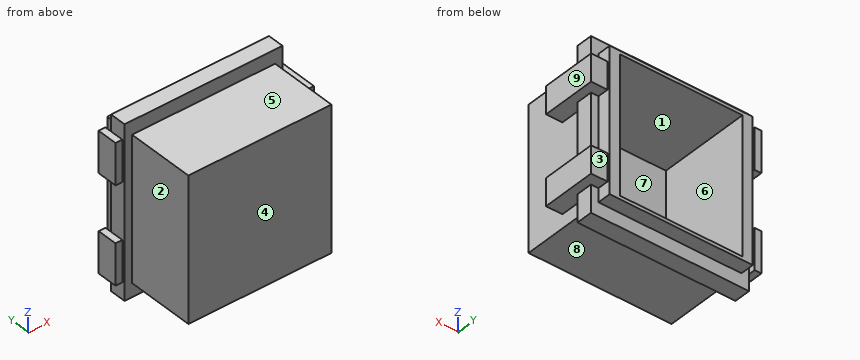
from build123d import *

# Parameters (mm, degrees)
SKETCH1_W           = 133.35
SKETCH1_H           = 133.35
BOSS_EXTRUDE1_DEPTH = 63.5
SKETCH2_W           = 147.32
SKETCH2_H           = 158.75
BOSS_EXTRUDE2_DEPTH = 15.24
SKETCH3_W           = 133.35
SKETCH3_H           = 133.35
BOSS_EXTRUDE3_DEPTH = 12.7
SKETCH4_W           = 38.1
SKETCH4_H           = 19.05
BOSS_EXTRUDE4_DEPTH = 6.35
SKETCH5_W           = 25.4
SKETCH5_H           = 50.8
BOSS_EXTRUDE5_DEPTH = 15.24
SKETCH7_W           = 114.3
SKETCH7_H           = 127
CUT_EXTRUDE1_DEPTH  = 86.36


with BuildPart() as part:
    # Sketch1 → Boss-Extrude1 (new body)
    with BuildSketch(Plane(origin=(0, 0, 0), x_dir=(1, 0, 0), z_dir=(0, 1, 0))):
        Rectangle(SKETCH1_W, SKETCH1_H)
    extrude(amount=BOSS_EXTRUDE1_DEPTH)

    # Sketch2 → Boss-Extrude2 (add)
    with BuildSketch(Plane(origin=(0, 63.5, 0), x_dir=(1, 0, 0), z_dir=(0, 1, 0))):
        Rectangle(SKETCH2_W, SKETCH2_H)
    extrude(amount=BOSS_EXTRUDE2_DEPTH)

    # Sketch3 → Boss-Extrude3 (add)
    with BuildSketch(Plane(origin=(0, 78.74, 0), x_dir=(1, 0, 0), z_dir=(0, 1, 0))):
        Rectangle(SKETCH3_W, SKETCH3_H)
    extrude(amount=BOSS_EXTRUDE3_DEPTH)

    # Sketch4 → Boss-Extrude4 (add)
    with BuildSketch(Plane.ZY.offset(73.66)):
        with Locations((45.085, 75.565)):
            Rectangle(SKETCH4_W, SKETCH4_H)
    boss_extrude4 = extrude(amount=BOSS_EXTRUDE4_DEPTH)

    # Mirror1: Boss-Extrude4 across plane
    add(boss_extrude4.mirror(Plane.XY))

    # Sketch5 → Boss-Extrude5 (add)
    with BuildSketch(Plane(origin=(66.675, 0, 0), x_dir=(0, 0, -1), z_dir=(1, 0, 0))):
        with Locations((-41.275, 63.5)):
            Rectangle(SKETCH5_W, SKETCH5_H)
    boss_extrude5 = extrude(amount=BOSS_EXTRUDE5_DEPTH)

    # Mirror2: Boss-Extrude5 across plane
    add(boss_extrude5.mirror(Plane.XY))

    # Sketch7 → Cut-Extrude1 (cut)
    with BuildSketch(Plane(origin=(0, 91.44, 0), x_dir=(1, 0, 0), z_dir=(0, 1, 0))):
        Rectangle(SKETCH7_W, SKETCH7_H)
    extrude(amount=-CUT_EXTRUDE1_DEPTH, mode=Mode.SUBTRACT)


solid = part.part
CAD build for the part. Positions are in the model's coordinates, mm. Face numbers are marked on the shaded views. A direction names the side the tool comes from. Coordinates: 2 decimals unless noted, no trailing zeros. Order: outer loops, then holes, each group sorted by start corner. A loop starts at its lowest first (then second) coordinate and runs counter-clockwise, first axis right, second up.
Item 1: Two-plate mould, pull along Z, no slides. Class the marked faces 6, 7, 8 and 9: +Z half, -Z half, draft (parallel to the pull), parting line (faces both ways), or undercut.
Check sheet entries:
face 6: undercut
face 7: undercut
face 8: -Z half
face 9: draft
Item 2: 3-axis set-ups, long thin cutter, end or side, ignore diameter. For the marked faces 1, 2, 3, 4 and 5: which of +Z, -Z, +X, -X, +Y, -Y reach the whole face in a straight line?
Check sheet entries:
face 1: +Y
face 2: +Z, -Z, -X, -Y
face 3: +Z, -Z, +X, +Y
face 4: +Z, -Z, +X, -X, -Y
face 5: +Z, +X, -X, -Y
Item 3: Drill centre lines: L1, parallel to X at y = 18.5, z = -17 (3 decimals); L2, parallel to X at y = 44.5, z = 40 (3 decimals); L3, parallel to Z at x = 53.5, y = 63 (3 decimals). Where is each one in solid material? Low to high.
Check sheet entries:
L1: x = -66.675 to -57.15, 57.15 to 66.675
L2: x = -66.675 to -57.15, 57.15 to 81.915
L3: z = -66.675 to -63.5, 63.5 to 66.675
Item 4: Pin check, flat tips, straight feed: pin 1 Ø2 at (x, z) = (69, -2) entering from -Y; pin 2 Ø5 at (x, y) = (-22, 18.5) entering from +Z (3 decimals); pin 3 Ø3 at (x, y) = (-18.5, 53.5) entering from -Z (3 decimals). Stop position of each tip, or through.
Check sheet entries:
pin 1: stops at y = 63.5
pin 2: stops at z = 66.675
pin 3: stops at z = -66.675
Item 5: Band-saw the part on D-D on z = -3. List the corners of the cut face in (x, y) (3 decimals), plus the area to 3 significant figures.
Check sheet entries:
outline: (-73.66, 63.5) - (-66.675, 63.5) - (-66.675, 0) - (66.675, 0) - (66.675, 63.5) - (73.66, 63.5) - (73.66, 78.74) - (66.675, 78.74) - (66.675, 91.44) - (57.15, 91.44) - (57.15, 5.08) - (-57.15, 5.08) - (-57.15, 91.44) - (-66.675, 91.44) - (-66.675, 78.74) - (-73.66, 78.74) - close
area: 2,540 mm2
Item 6: Band-saw the part on A-A on y = 13.5. List the corners of the cut face in (x, z) (3 decimals), plus the area to 3 significant figures.
Check sheet entries:
outline: (-66.675, -66.675) - (66.675, -66.675) - (66.675, 66.675) - (-66.675, 66.675) - close; hole (-57.15, -63.5) - (57.15, -63.5) - (57.15, 63.5) - (-57.15, 63.5) - close
area: 3,270 mm2
Item 7: Band-saw the part on B-B on z = 39. List the corners of the cut face in (x, y) (3 decimals).
Check sheet entries:
outline: (-80.01, 66.04) - (-73.66, 66.04) - (-73.66, 63.5) - (-66.675, 63.5) - (-66.675, 0) - (66.675, 0) - (66.675, 38.1) - (81.915, 38.1) - (81.915, 88.9) - (66.675, 88.9) - (66.675, 91.44) - (57.15, 91.44) - (57.15, 5.08) - (-57.15, 5.08) - (-57.15, 91.44) - (-66.675, 91.44) - (-66.675, 78.74) - (-73.66, 78.74) - (-73.66, 85.09) - (-80.01, 85.09) - close
Item 8: Band-saw the part on C-C on x = -50.5. List the corners of the cut face in (y, z) (3 decimals), plus the area to 3 significant figures.
Check sheet entries:
outline: (0, -66.675) - (63.5, -66.675) - (63.5, -79.375) - (78.74, -79.375) - (78.74, -66.675) - (91.44, -66.675) - (91.44, -63.5) - (5.08, -63.5) - (5.08, 63.5) - (91.44, 63.5) - (91.44, 66.675) - (78.74, 66.675) - (78.74, 79.375) - (63.5, 79.375) - (63.5, 66.675) - (0, 66.675) - close
area: 1,610 mm2
